Build history of the part. All positions in model axes, mm. Round coordinates to 2 decimals unless told otherwise and drop trailing zeros. Write each loop counter-clockwise with the first axis right and the second up, starting at its lowest first coordinate (ties: lowest second). Pieces come first, ordered by that corner, then holes. Notation, with made-up numbers: (-16, -3.75) - (7, -3.75) arc R12 cw to (7, 9.25) - close; hole circle Ø4 at (-8, -29.75). An arc over 180 degrees is marked (long way). Write each question's results on one line, items separated by ' | '.
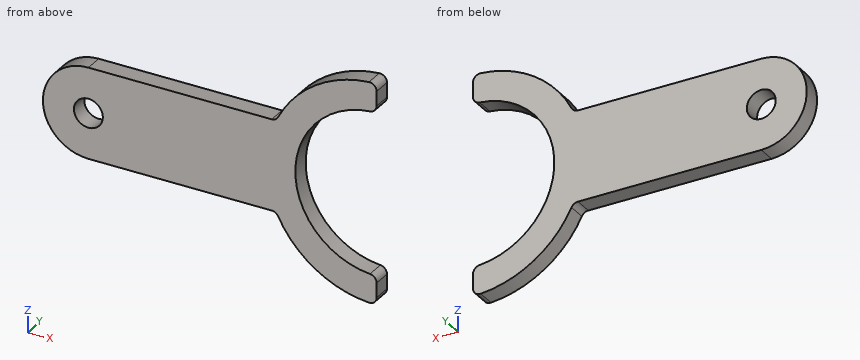
from build123d import *

# Parameters (mm, degrees)
SKETCH1_R           = 4
BOSS_EXTRUDE1_DEPTH = 5


with BuildPart() as part:
    # Sketch1 → Boss-Extrude1 (new body)
    with BuildSketch(Plane(origin=(0, 0, 0), x_dir=(1, 0, 0), z_dir=(0, 1, 0))):
        with BuildLine():
            Line((0, 12.580465515), (50.714293016, 12.580465515))
            ThreePointArc((50.714293016, 12.580465515), (51.764359173, 12.878301873), (52.501677451, 13.68310445))
            ThreePointArc((52.501677451, 13.68310445), (62.84292145, 25.376627415), (77.615630991, 30.421115454))
            ThreePointArc((77.615630991, 30.421115454), (79.119682878, 29.889047403), (79.756, 28.4260474))
            Line((79.756, 28.4260474), (79.756, 24.418230894))
            ThreePointArc((79.756, 24.418230894), (79.226804306, 23.06296904), (77.919265306, 22.424905923))
            ThreePointArc((77.919265306, 22.424905923), (57.256, 0), (77.919265306, -22.424905923))
            ThreePointArc((77.919265306, -22.424905923), (79.226804306, -23.06296904), (79.756, -24.418230894))
            Line((79.756, -24.418230894), (79.756, -28.4260474))
            ThreePointArc((79.756, -28.4260474), (79.119682878, -29.889047403), (77.615630991, -30.421115454))
            ThreePointArc((77.615630991, -30.421115454), (62.84292145, -25.376627415), (52.501677451, -13.68310445))
            ThreePointArc((52.501677451, -13.68310445), (51.764359173, -12.878301873), (50.714293016, -12.580465515))
            Line((50.714293016, -12.580465515), (0, -12.580465515))
            ThreePointArc((0, -12.580465515), (-12.580465515, 0), (0, 12.580465515))
        make_face()
        with Locations(Location((0, 0, 0), (0, 0, 270))):
            Circle(SKETCH1_R, mode=Mode.SUBTRACT)
    extrude(amount=BOSS_EXTRUDE1_DEPTH)


solid = part.part
(1) Slice it at A-A, the plane z = 0. Write the cut outline in (x, y), and give its area (3 significant figures).
Worked answers:
outline: (-12.58, 0) - (-4, 0) - (-4, 5) - (-12.58, 5) - close; (4, 0) - (57.26, 0) - (57.26, 5) - (4, 5) - close | area: 309 mm2
(2) Slice it at D-D, the plane z = -8. Write the cut outline in (x, y).
Worked answers:
outline: (-9.71, 0) - (58.73, 0) - (58.73, 5) - (-9.71, 5) - close
(3) Drill centre lines: probe 1 along X at (y, z) = (1.3, 0); probe 2 along Z at (x, y) = (75.5, 4.8); probe 3 along Z at (x, y) = (39, 1.4). Where is each one in solid material? Low to high. Write a range as [from, to].
Worked answers:
probe 1: x = [-12.58, -4], [4, 57.26] | probe 2: z = [-30.2, -22.09], [22.09, 30.2] | probe 3: z = [-12.58, 12.58]
(4) Slice it at B-B, the plane y = 2.2. Write the cut outline in (x, z), and give its area (3 significant figures).
Worked answers:
outline: (0, -12.58) - (50.71, -12.58) arc R2 cw to (52.5, -13.68) arc R30.5 ccw to (77.62, -30.42) arc R2 ccw to (79.76, -28.43) - (79.76, -24.42) arc R2 ccw to (77.92, -22.42) arc R22.5 cw to (77.92, 22.42) arc R2 ccw to (79.76, 24.42) - (79.76, 28.43) arc R2 ccw to (77.62, 30.42) arc R30.5 ccw to (52.5, 13.68) arc R2 cw to (50.71, 12.58) - (0, 12.58) arc R12.58 ccw to start; hole circle Ø8 at (0, 0) | area: 2,120 mm2
(5) Slice it at C-C, the plane z = 15.5. Write the cut outline in (x, y).
Worked answers:
outline: (53.49, 0) - (63.45, 0) - (63.45, 5) - (53.49, 5) - close
(6) Flat gauge pins, fed straight in: pin 1 Ø1.5 at (y, z) = (0.5, -2.5) entering from +X; pin 2 Ø1 at (y, z) = (1.5, 7.5) entering from -X. Where does each tip first touch, or does it go through?
Worked answers:
pin 1: stops at x = 57.49 | pin 2: stops at x = -10.45
